Model file for the job. Use its own axes, mm. A direction names the side the tool comes from. Round coordinates to 2 decimals unless told otherwise and drop trailing zeros. Write each loop counter-clockwise with the first axis right and the second up, starting at its lowest first coordinate (ties: lowest second). Pieces come first, ordered by that corner, then holes. Notation, with made-up numbers: (10.5, 85) - (33.5, 85) arc R22 cw to (33.5, 120) - close; hole circle Ø3 at (29, 47.25). An arc over 180 degrees is marked (long way). One line per item, written item: value.
Autodesk Inventor part; units mm, degrees
ref_plane "YZ Plane" through (0, 0, 0) normal (1, 0, 0) x (0, 1, 0)
ref_plane "XZ Plane" through (0, 0, 0) normal (0, 1, 0) x (-1, 0, 0)
ref_plane "XY Plane" through (0, 0, 0) normal (0, 0, 1) x (1, 0, 0)
sketch "Sketch1" plane through (0, 0, 0) normal (0, 1, 0) x (-1, 0, 0)
  arc A0 (6.4507, -0.7992) -> (-6.4507, -0.7992) centre (0, 0) ccw
  arc A1 (-3.4734, -24.8303) -> (3.4734, -24.8303) centre (0, -24.4) ccw
  line L0 (0, -34.78) -> (0, 13.38)
  line L1 (6.4507, -0.7992) -> (3.4734, -24.8303)
  line L2 (-6.4507, -0.7992) -> (-3.4734, -24.8303)
  circle A2 centre (0, -22.9) radius 1.5
  dimension "d0" = 13
  dimension "d1" = 7
  dimension "d2" = 34.4
  dimension "d3" = 3
  dimension "d4" = 1.5
extrude "Extrusion1" add sketch "Sketch1" along normal blind 3 contours L1 A1 L0 A2 A0 | L0 A2 A1 L2 A0
sketch "Sketch2" plane through (0, 3, 0) normal (0, 1, 0) x (1, 0, 0)
  circle A0 centre (0, 0) radius 4.675
  dimension "d7" = 9.35
extrude "Extrusion2" add sketch "Sketch2" along normal blind 5
sketch "Sketch3" plane through (0, 8, 0) normal (0, 1, 0) x (1, 0, 0)
  circle A0 centre (0, 0) radius 3
  dimension "d10" = 6
extrude "Extrusion3" cut sketch "Sketch3" against normal blind 2.5
sketch "Sketch4" plane through (0, 0, 0) normal (0, -1, 0) x (1, 0, 0)
  circle A0 centre (0, 0) radius 6
  dimension "d13" = 12
extrude "Extrusion4" add sketch "Sketch4" along normal blind 1
fillet "Fillet1" radius 0.5 1 edges at (-6, -1, 0)
sketch "Sketch5" plane through (0, -1, 0) normal (0, -1, 0) x (1, 0, 0)
  circle A0 centre (0, 0) radius 3
  dimension "d17" = 6
extrude "Extrusion5" cut sketch "Sketch5" against normal blind 4
sketch "Sketch6" plane through (0, 3, 0) normal (0, -1, 0) x (1, 0, 0)
  circle A0 centre (0, 0) radius 2
  dimension "d20" = 4
extrude "Extrusion6" cut sketch "Sketch6" against normal through all
properties part number "RCT-P070_servo_linkage"
1. Band-saw the part on B-B on x = 0. State how many separate pieces and enclosed holes the cut face has, plus the area to 3 significant figures.
Report:
separate pieces: 3
enclosed holes: 0
area: 104 mm²
2. Tool access for faces 5 (the face through (0, 4, -2)), 6 (the face through (-1.013, 5.465, -4.564)), 7 (the face through (1, 3, -2)): list every direction of +Z, -Z, +X, -X, +Y, -Y with a clear straight run to the whole face (end or side of a thin tool).
Report:
face 5: +Y, -Y
face 6: +Y
face 7: -Y
3. Band-saw the part on A-A on z = 0. Write the cut outline in (x, y) (3 decimals).
Report:
outline: (-6.5, 0) - (-6, 0) - (-6, -0.5) arc R0.5 ccw to (-5.5, -1) - (-3, -1) - (-3, 3) - (-2, 3) - (-2, 5.5) - (-3, 5.5) - (-3, 8) - (-4.675, 8) - (-4.675, 3) - (-6.5, 3) - close; (2, 3) - (3, 3) - (3, -1) - (5.5, -1) arc R0.5 ccw to (6, -0.5) - (6, 0) - (6.5, 0) - (6.5, 3) - (4.675, 3) - (4.675, 8) - (3, 8) - (3, 5.5) - (2, 5.5) - close
4. Wall check: probe 1 along Z at (x, y) = (0, 1.15); probe 2 along X at (y, z) = (6.8, 0) (3 decimals). Give the ranges that are in metal, low to high. Write a range as [from, to].
Report:
probe 1: [-27.9, -24.4], [-21.4, -3], [3, 6.5]
probe 2: [-4.675, -3], [3, 4.675]
5. Mould opens along Z. For faces 1 (the face through (-4.983, 1.479, -12.647)), 2 (the face through (0, 0, -14)), 3 (the face through (1, 5.5, 2)), 4 (the face through (-3, 7, 0)) say: released by +Z, released by -Z, zero draft, split by the parting line, or undercut.
Report:
face 1: released by -Z
face 2: zero draft
face 3: undercut
face 4: undercut
6. Drop flat-ended pins along their axis: pin 1 (6.5 mm diameter, centred on x = 0.5, z = 0.5, fed in from -Y); pin 2 (1 mm diameter, centred on x = -4, z = -18, fed in from -Y); pin 3 (5 mm diameter, centred on x = 0, z = 0, fed in from +Y); pin 4 (3 mm diameter, centred on x = 2, y = 0.5, fed in from +Z). Give the stop position or say it passes through.
Report:
pin 1: y = -1
pin 2: y = 0
pin 3: y = 5.5
pin 4: z = 6.48
7. Band-saw the part on D-D on y = 6. Write the cut outline in (x, z) (3 decimals), plus the area to 3 significant figures.
Report:
outline: circle Ø9.35 at (0, 0); hole circle Ø6 at (0, 0)
area: 40.4 mm²
8. Band-saw the part on C-C on y = 1.25. Write the cut outline in (x, z).
Report:
outline: (-6.45, -0.8) - (-3.47, -24.83) arc R3.5 ccw to (3.47, -24.83) - (6.45, -0.8) arc R6.5 ccw (long way) to start; hole circle Ø6 at (0, 0); hole circle Ø3 at (0, -22.9)
